Source: CAD feature listing. Evaluate the final solid. Frame: model axes, mm. Give positions to 0.01 mm unless a question says otherwise; leave off trailing zeros. Order: outer loops, then holes, each group sorted by start corner. A loop starts at its lowest first (then second) coordinate and runs counter-clockwise, first axis right, second up. Notation, with made-up numbers: M 8.5,29 L 21.5,29 A13 ccw 21.5,49 Z; hole C 46,-12.75 d3. An arc over 180 degrees is marked long. Answer in a Markdown table with one row per item. Add a question column.
(1) Pin query (flat end, axial travel): P1, Ø0.5, axis at y = 5.5, z = 16.5, coming from the -X side (3 decimals); P2, Ø0.5, axis at x = -7, y = 5.5, coming from the +Z side (3 decimals); P3, Ø0.5, axis at x = 18, y = 5.5, coming from the -Z side (3 decimals). Return the tip coordinate at first contact, or that it passes through.
(2) Section query B-B, the plane x = 19. Return loops of the section in (y, z) (3 decimals), plus the area to 3 significant figures.
(3) Mould query, pull axis X, two halves, no side actions, for faces 1 (the face through (-23.5, 2, 0)), 2 (the face through (-6, 7, -1)), 3 (the face through (0, 5, 4)). Classes: pulls with the +X half, pulls with the -X half, needs draft (parallel to the pull), parting line crosses it, or undercut.
(4) Section query C-C, the plane x = -11.5. Return loops of the section in (y, z), plus the area to 3 significant figures.
(5) Section query A-A, the plane z = 19. Return loops of the section in (x, y) (3 decimals).
(6) Material intervals for line 1 along Z through (x, y) = (-7, 5.5) (3 decimals); line 2 along Z through (x, y) = (-10, 6.25); line 3 along Y through (x, z) = (-11.5, -7), sorted ascending.
(7) Section query D-D, the plane z = -10.5. Return loops of the section in (x, y), plus the area to 3 significant figures.
from build123d import *

# Parameters (mm, degrees)
SKETCH1_W              = 47
SKETCH1_H              = 49
BOSS_EXTRUDE1_DEPTH    = 5
SKETCH2_W              = 9
SKETCH2_H              = 12
BOSS_EXTRUDE2_DEPTH    = 2
FILLET1_R              = 1
LPATTERN1_COUNT        = 4
LPATTERN1_PITCH        = 11.75
LPATTERN1_COUNT_DIR2   = 3
LPATTERN1_PITCH_DIR2   = 17
FILLET1_OF_LPATTERN1_R = 1


with BuildPart() as part:
    # Sketch1 → Boss-Extrude1 (new body)
    with BuildSketch(Plane(origin=(0, 0, 0), x_dir=(1, 0, 0), z_dir=(0, 1, 0))):
        Rectangle(SKETCH1_W, SKETCH1_H)
    extrude(amount=BOSS_EXTRUDE1_DEPTH)

    # Sketch2 → Boss-Extrude2 (add)
    with BuildSketch(Plane(origin=(0, 5, 0), x_dir=(1, 0, 0), z_dir=(0, 1, 0))):
        with Locations((-17.625, 17.625)):
            Rectangle(SKETCH2_W, SKETCH2_H)
    boss_extrude2 = extrude(amount=BOSS_EXTRUDE2_DEPTH)

    # Fillet1
    fillet1_edges = [part.edges().sort_by_distance(p)[0] for p in [
        (-13.125, 7, -17.625),
        (-17.625, 7, -23.625),
        (-17.625, 7, -11.625),
        (-22.125, 7, -17.625),
    ]]
    fillet(fillet1_edges, radius=FILLET1_R)

    # LPattern1: Boss-Extrude2 4 × 3
    with Locations(*[(i * LPATTERN1_PITCH, 0, j * LPATTERN1_PITCH_DIR2) for i in range(LPATTERN1_COUNT) for j in range(LPATTERN1_COUNT_DIR2) if (i, j) != (0, 0)]):
        add(boss_extrude2)

    # Fillet1 of LPattern1
    fillet1_of_lpattern1_edges = [part.edges().sort_by_distance(p)[0] for p in [
        (-13.125, 7, -0.625),
        (-17.625, 7, -6.625),
        (-17.625, 7, 5.375),
        (-22.125, 7, -0.625),
        (-13.125, 7, 16.375),
        (-17.625, 7, 10.375),
        (-17.625, 7, 22.375),
        (-22.125, 7, 16.375),
        (-1.375, 7, -17.625),
        (-5.875, 7, -23.625),
        (-5.875, 7, -11.625),
        (-10.375, 7, -17.625),
        (-1.375, 7, -0.625),
        (-5.875, 7, -6.625),
        (-5.875, 7, 5.375),
        (-10.375, 7, -0.625),
        (-1.375, 7, 16.375),
        (-5.875, 7, 10.375),
        (-5.875, 7, 22.375),
        (-10.375, 7, 16.375),
        (10.375, 7, -17.625),
        (5.875, 7, -23.625),
        (5.875, 7, -11.625),
        (1.375, 7, -17.625),
        (10.375, 7, -0.625),
        (5.875, 7, -6.625),
        (5.875, 7, 5.375),
        (1.375, 7, -0.625),
        (10.375, 7, 16.375),
        (5.875, 7, 10.375),
        (5.875, 7, 22.375),
        (1.375, 7, 16.375),
        (22.125, 7, -17.625),
        (17.625, 7, -23.625),
        (17.625, 7, -11.625),
        (13.125, 7, -17.625),
        (22.125, 7, -0.625),
        (17.625, 7, -6.625),
        (17.625, 7, 5.375),
        (13.125, 7, -0.625),
        (22.125, 7, 16.375),
        (17.625, 7, 10.375),
        (17.625, 7, 22.375),
        (13.125, 7, 16.375),
    ]]
    fillet(fillet1_of_lpattern1_edges, radius=FILLET1_OF_LPATTERN1_R)


solid = part.part
Values follow:
| question | item | result |
|---|---|---|
| 1 | P1 | stops at x = -22.125 |
| 1 | P2 | stops at z = 22.375 |
| 1 | P3 | stops at z = -23.625 |
| 2 | outline | M 0,-24.5 L 5,-24.5 L 5,-23.625 L 6,-23.625 A1 ccw 7,-22.625 L 7,-12.625 A1 ccw 6,-11.625 L 5,-11.625 L 5,-6.625 L 6,-6.625 A1 ccw 7,-5.625 L 7,4.375 A1 ccw 6,5.375 L 5,5.375 L 5,10.375 L 6,10.375 A1 ccw 7,11.375 L 7,21.375 A1 ccw 6,22.375 L 5,22.375 L 5,24.5 L 0,24.5 Z |
| 2 | area | 316 mm² |
| 3 | face 1 | pulls with the -X half |
| 3 | face 2 | needs draft |
| 3 | face 3 | undercut |
| 4 | outline | M 0,-24.5 L 5,-24.5 L 5,24.5 L 0,24.5 Z |
| 4 | area | 245 mm² |
| 5 | outline | M -23.5,0 L 23.5,0 L 23.5,5 L 22.125,5 L 22.125,6 A1 ccw 21.125,7 L 14.125,7 A1 ccw 13.125,6 L 13.125,5 L 10.375,5 L 10.375,6 A1 ccw 9.375,7 L 2.375,7 A1 ccw 1.375,6 L 1.375,5 L -1.375,5 L -1.375,6 A1 ccw -2.375,7 L -9.375,7 A1 ccw -10.375,6 L -10.375,5 L -13.125,5 L -13.125,6 A1 ccw -14.125,7 L -21.125,7 A1 ccw -22.125,6 L -22.125,5 L -23.5,5 Z |
| 6 | line 1 | z = -23.625 to -11.625, -6.625 to 5.375, 10.375 to 22.375 |
| 6 | line 2 | z = -23.59 to -11.66, -6.59 to 5.34, 10.41 to 22.34 |
| 6 | line 3 | y = 0 to 5 |
| 7 | outline | M -23.5,0 L 23.5,0 L 23.5,5 L -23.5,5 Z |
| 7 | area | 235 mm² |
